Check sheet for the modelled part. Datum: model origin and axes. Units: mm. A direction names the side the tool comes from. Give positions to 0.01 mm unless a question says otherwise; leave off trailing zeros. Order: outer loops, then holes, each group sorted by start corner. A loop starts at its lowest first (then second) coordinate and runs counter-clockwise, first axis right, second up. Notation, with made-up numbers: (31.5, 7.5) -> (63.5, 7.5) arc R11 ccw to (63.5, 15.5) -> close; hole circle Ø3 at (45.5, 78.25). An arc over 180 degrees is marked (long way). Answer in a Markdown table with one row per item. Add a question column.
(1) Set-up check for faces 4 (the face through (15, -1, 45)), 5 (the face through (10, -55, 1)): record each of +Z, -Z, +X, -X, +Y, -Y from which the full face is reachable in a straight line by a thin tool's end or side.
(2) Thickness scan on L1, parallel to Y at x = 20.25, z = 44.5; L2, parallel to Z at x = 15.5, y = 20; L3, parallel to X at y = 51.7, z = 0. Record the ranges inside material, lowest first. Write a range as [from, to].
(3) Cross-section at B-B (z = 0). Record the cut outline in (x, y).
(4) Go/stop test with a flat-tipped pin: pin 1 (12 mm diameter, centred on y = 30, z = 16, fed in from +X). Record where the tip stops, or that it passes through.
(5) Cross-section at C-C (y = 0). Record the cut outline in (x, z), then the cut area to 3 significant figures.
(6) Cross-section at D-D (x = 7.75). Record the cut outline in (y, z), then the cut area to 3 significant figures.
(7) Cross-section at A-A (x = 17.16). Record the cut outline in (y, z), then the cut area to 3 significant figures.
(8) Release check for a two-part mould opening along X. For faces 1 (the face through (25, 0, 48)), 2 (the face through (24.1, -52.5, 0.9)), 3 (the face through (12, -1, 50)) record: released by +X, released by -X, zero draft, split by the parting line, or undercut.
```python
from build123d import *

# Parameters (mm, degrees)
SKETCH2_W           = 100
SKETCH2_H           = 110
SKETCH2_W_2         = 90
SKETCH2_H_2         = 100
BOSS_EXTRUDE1_DEPTH = 5
SKETCH2_3_W         = 100
SKETCH2_3_H         = 110
SKETCH2_3_W_2       = 90
SKETCH2_3_H_2       = 100
BOSS_EXTRUDE2_DEPTH = 25
SKETCH3_R           = 7
CUT_EXTRUDE1_DEPTH  = 124.389626793


with BuildPart() as part:
    # Sketch2 → Boss-Extrude1 (new body)
    with BuildSketch(Plane(origin=(0, 0, 0), x_dir=(0, 0, -1), z_dir=(1, 0, 0))):
        Rectangle(SKETCH2_W, SKETCH2_H)
        Rectangle(SKETCH2_W_2, SKETCH2_H_2, mode=Mode.SUBTRACT)
        Rectangle(SKETCH2_W_2, SKETCH2_H_2)
    extrude(amount=BOSS_EXTRUDE1_DEPTH)

    # Sketch2_3 → Boss-Extrude2 (add)
    with BuildSketch(Plane(origin=(0, 0, 0), x_dir=(0, 0, -1), z_dir=(1, 0, 0))):
        Rectangle(SKETCH2_3_W, SKETCH2_3_H)
        Rectangle(SKETCH2_3_W_2, SKETCH2_3_H_2, mode=Mode.SUBTRACT)
    extrude(amount=BOSS_EXTRUDE2_DEPTH)

    # Sketch3 → Cut-Extrude1 (cut, through all)
    with BuildSketch(Plane.XZ.offset(55)):
        with Locations(Location((17.16, 0, 0), (0, 0, 270))):
            Circle(SKETCH3_R)
    extrude(amount=-CUT_EXTRUDE1_DEPTH, mode=Mode.SUBTRACT)


solid = part.part
```
Answer below:
| question | item | result |
|---|---|---|
| 1 | face 4 | +X |
| 1 | face 5 | +Z, -Z, +X, -X, -Y |
| 2 | L1 | y = [-55, -50], [50, 55] |
| 2 | L2 | z = [-50, -45], [45, 50] |
| 2 | L3 | x = [0, 10.16], [24.16, 25] |
| 3 | outline | (0, -55) -> (10.16, -55) -> (10.16, -50) -> (5, -50) -> (5, 50) -> (10.16, 50) -> (10.16, 55) -> (0, 55) -> close; (24.16, -55) -> (25, -55) -> (25, -50) -> (24.16, -50) -> close; (24.16, 50) -> (25, 50) -> (25, 55) -> (24.16, 55) -> close |
| 4 | pin 1 | stops at x = 5 |
| 5 | outline | (0, -50) -> (25, -50) -> (25, -45) -> (5, -45) -> (5, 45) -> (25, 45) -> (25, 50) -> (0, 50) -> close |
| 5 | area | 700 mm² |
| 6 | outline | (-55, -50) -> (55, -50) -> (55, 50) -> (-55, 50) -> close; hole (-50, -45) -> (50, -45) -> (50, 45) -> (-50, 45) -> close |
| 6 | area | 2,000 mm² |
| 7 | outline | (-55, -50) -> (55, -50) -> (55, -7) -> (50, -7) -> (50, -45) -> (-50, -45) -> (-50, -7) -> (-55, -7) -> close; (-55, 7) -> (-50, 7) -> (-50, 45) -> (50, 45) -> (50, 7) -> (55, 7) -> (55, 50) -> (-55, 50) -> close |
| 7 | area | 1,860 mm² |
| 8 | face 1 | released by +X |
| 8 | face 2 | undercut |
| 8 | face 3 | zero draft |
